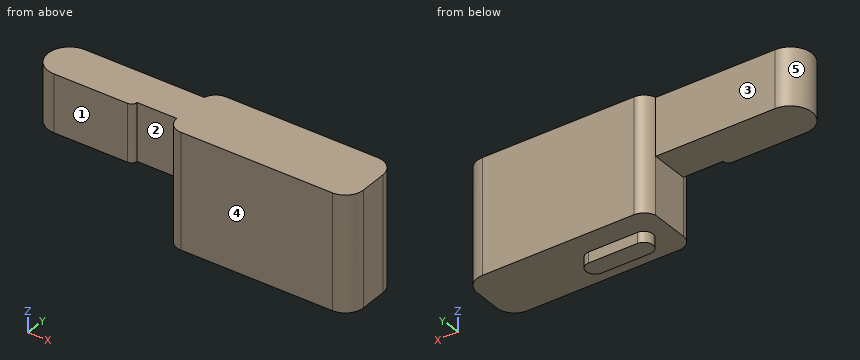
from build123d import *

# Parameters (mm, degrees)
F1_DEPTH = 32
F2_DEPTH = 16
F4_DEPTH = 3


with BuildPart() as f1:
    # F0 (on Top) → F1 (new body)
    with BuildSketch(Plane.XY):
        with BuildLine():
            Line((21.5, 8.75), (-20.5, 8.75))
            ThreePointArc((-20.5, 8.75), (-22.94949, 7.912278), (-24.372983, 5.75))
            Line((-24.372983, 5.75), (-24.5, -4.75))
            ThreePointArc((-24.5, -4.75), (-23.328427, -7.578427), (-20.5, -8.75))
            Line((-20.5, -8.75), (21.5, -8.75))
            ThreePointArc((21.5, -8.75), (25.035534, -7.285534), (26.5, -3.75))
            Line((26.5, -3.75), (26.5, 3.75))
            ThreePointArc((26.5, 3.75), (25.035534, 7.285534), (21.5, 8.75))
        make_face()
    extrude(amount=-F1_DEPTH)

    # F0 (on Top) → F2 (join)
    with BuildSketch(Plane.XY):
        with BuildLine():
            Line((-24.5, -4.75), (-24.372983, 5.75))
            Line((-24.372983, 5.75), (-57.372983, 5.75))
            ThreePointArc((-57.372983, 5.75), (-63.372983, -0.25), (-57.372983, -6.25))
            Line((-57.372983, -6.25), (-37, -6.25))
            ThreePointArc((-37, -6.25), (-35.93934, -5.81066), (-35.5, -4.75))
            Line((-35.5, -4.75), (-24.5, -4.75))
        make_face()
    extrude(amount=-F2_DEPTH)

    # F3 (on face) → F4 (join)
    with BuildSketch(Plane(origin=(0, 0, -32), x_dir=(1, 0, 0), z_dir=(0, 0, -1))):
        with BuildLine():
            ThreePointArc((-3.5, -2.5), (-1, 0), (-3.5, 2.5))
            Line((-3.5, 2.5), (-17, 2.5))
            ThreePointArc((-17, 2.5), (-19.5, 0), (-17, -2.5))
            Line((-17, -2.5), (-3.5, -2.5))
        make_face()
    extrude(amount=F4_DEPTH)


solid = f1.part
Can you work these out from the model? Positions are in its coordinate system, mm. Face numbers are marked on the shaded views. A direction names the side the tool comes from. Round coordinates to 2 decimals unless told otherwise and drop trailing zeros. Loops run counter-clockwise (first coordinate to the right, second up) from the corner with the lowest first, then second, coordinate; pieces in that order, holes last. Notation, with made-up numbers: (76, 4.25) - (101, 4.25) arc R15 cw to (101, 9.25) - close; hole circle Ø6 at (1.5, 52). An arc over 180 degrees is marked (long way). Use CSV: the item, a comma, the result in double quotes. Start each with the question number.
1) For the marked faces 1, 2, 3, 4 and 5, which set-ups out of +Z, -Z, +X, -X, +Y, -Y let a thin tool reach every point of the face, with its end or its side?
2) If we section it at D-D on z = -30: Write out the boundary of the cut face in (x, y).
3) If we section it at C-C on y = 0: Write out the boundary of the cut face in (x, z).
4) If we section it at B-B on x = 10: Write out the boundary of the cut face in (y, z).
5) If we section it at A-A on z = -9: Write out the boundary of the cut face in (x, y).
6) For pin 1 Ø5 at (y, z) = (6.5, -31) entering from -X; pin 2 Ø5 at (x, y) = (-12.5, -4.5) entering from +Z; pin 3 Ø4 at (x, z) = (-23, -20.5) entering from -Y; pin 4 Ø3 at (x, y) = (-6.5, -6) entering from -Z, each with a flat end and sliding along its axis, tell me the tip position at first contact or that it passes through.
7) Please list where these lines run through material, in increasing order: probe 1 along Y at (x, z) = (-51, -15); probe 2 along Z at (x, y) = (6, 5); probe 3 along Z at (x, y) = (-46, -2). Write a range as [from, to].
Geometry results:
1,face 1,"+Z, -Z, -X, -Y"
1,face 2,"+Z, -Z, -Y"
1,face 3,"+Z, -Z, -X, +Y"
1,face 4,"+Z, -Z, +X, -X, -Y"
1,face 5,"+Z, -Z, -X"
2,outline,"(-24.5, -4.75) arc R4 ccw to (-20.5, -8.75) - (21.5, -8.75) arc R5 ccw to (26.5, -3.75) - (26.5, 3.75) arc R5 ccw to (21.5, 8.75) - (-20.5, 8.75) arc R4 ccw to (-24.37, 5.75) - close"
3,outline,"(-63.37, -16) - (-24.44, -16) - (-24.44, -32) - (-19.5, -32) - (-19.5, -35) - (-1, -35) - (-1, -32) - (26.5, -32) - (26.5, 0) - (-63.37, 0) - close"
4,outline,"(-8.75, -32) - (8.75, -32) - (8.75, 0) - (-8.75, 0) - close"
5,outline,"(-57.37, -6.25) - (-37, -6.25) arc R1.5 ccw to (-35.5, -4.75) - (-24.5, -4.75) arc R4 ccw to (-20.5, -8.75) - (21.5, -8.75) arc R5 ccw to (26.5, -3.75) - (26.5, 3.75) arc R5 ccw to (21.5, 8.75) - (-20.5, 8.75) arc R4 ccw to (-24.37, 5.75) - (-57.37, 5.75) arc R6 ccw to start"
6,pin 1,"stops at x = -24.39"
6,pin 2,"stops at z = 0"
6,pin 3,"stops at y = -8.72"
6,pin 4,"stops at z = -32"
7,probe 1,"y = [-6.25, 5.75]"
7,probe 2,"z = [-32, 0]"
7,probe 3,"z = [-16, 0]"
